Source: CAD feature listing. Evaluate the final solid. Frame: model axes, mm. Face numbers are marked on the shaded views. A direction names the side the tool comes from. Give positions to 0.01 mm unless a question says otherwise; leave off trailing zeros. Loops run counter-clockwise (first coordinate to the right, second up) from the corner with the lowest first, then second, coordinate; pieces in that order, holes last. Notation, with made-up numbers: M -33.5,72 L -21.5,72 A29 ccw -21.5,104 Z; hole C -13,52 d7. An arc over 180 degrees is marked long. Put each result on its own line as item: value. Start each with the question number.
Autodesk Inventor part; units mm, degrees
ref_plane "bolt_to_parts_XY" through (0, 0, 0) normal (1, 0, 0) x (0, 0, -1)
ref_plane "bolt_to_parts_YZ" through (0, 0, 0) normal (0, 0, -1) x (0, 1, 0)
ref_plane "bolt_to_parts_ZX" through (0, 0, 0) normal (0, 1, 0) x (1, 0, 0)
sketch "Sketch_1" plane through (0, 0, 0) normal (0, 0, 1) x (1, 0, 0)
  line L0 (5, 0) -> (-2.5, 0)
  line L1 (-2.5, 0) -> (-2.5, 0.94)
  arc A0 (0, 4.7) -> (-2.5, 0.94) centre (2.1827, 0.5376) ccw
  line L2 (0, 4.7) -> (0, 2)
  line L3 (0, 2) -> (4.5705, 2)
  line L4 (4.5705, 2) -> (5, 1.5705)
  line L5 (5, 1.5705) -> (5, 0)
  line L6 (5, 0) -> (-2.5, 0)
revolve "Revolution1" add sketch "Sketch_1" angle 360 about axis through (5, 0, 0) along (1, 0, 0)
thread "Thread1"
sketch "Sketch_2" plane through (-2.5, 0, 0) normal (1, 0, 0) x (0, 0, -1)
  line L0 (-2.35, 0.6267) -> (-2.35, -0.6267)
  line L1 (-2.35, -0.6267) -> (-0.6267, -0.6267)
  line L2 (-0.6267, -0.6267) -> (-0.6267, -2.35)
  line L3 (-0.6267, -2.35) -> (0.6267, -2.35)
  line L4 (0.6267, -2.35) -> (0.6267, -0.6267)
  line L5 (0.6267, -0.6267) -> (2.35, -0.6267)
  line L6 (2.35, -0.6267) -> (2.35, 0.6267)
  line L7 (2.35, 0.6267) -> (0.6267, 0.6267)
  line L8 (0.6267, 0.6267) -> (0.6267, 2.35)
  line L9 (0.6267, 2.35) -> (-0.6267, 2.35)
  line L10 (-0.6267, 2.35) -> (-0.6267, 0.6267)
  line L11 (-0.6267, 0.6267) -> (-2.35, 0.6267)
extrude "Extrusion1" cut sketch "Sketch_2" along normal mid plane 2.5
ref_plane "bolt_to_parts_XY" through (0, 0, 0) normal (1, 0, 0) x (0, 0, -1)
ref_plane "bolt_to_parts_YZ" through (0, 0, 0) normal (0, 0, -1) x (0, 1, 0)
ref_plane "bolt_to_parts_ZX" through (0, 0, 0) normal (0, 1, 0) x (1, 0, 0)
properties part number "BOX-TRSS4-5"
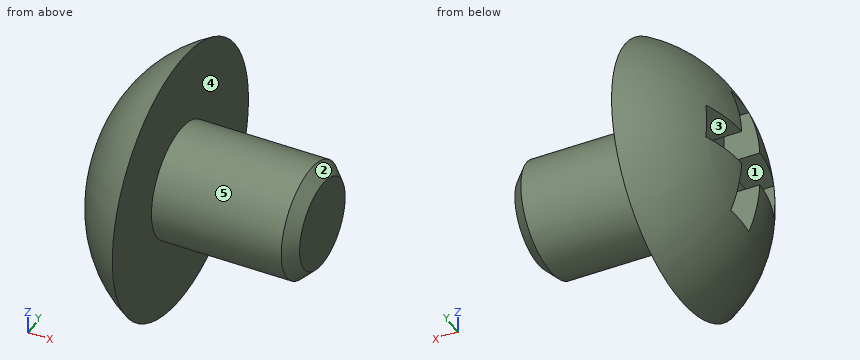
1. Section A-A, the plane x = 3. Output: boundary loops of the cut face in (y, z).
2. Ray query, line 1 (X direction, y = 1.25, z = 2); line 2 (X direction, y = 0, z = -0.5); line 3 (Z direction, x = 3.5, y = -0.25). Return the intervals inside material, ascending.
3. Set-up query: the marked faces 1 and 2. Return all of +Z, -Z, +X, -X, +Y, -Y with unobstructed straight access to the full face (end or side cutting, diameter ignored); none if empty.
4. Pull-direction query (Z, two-part tool) for the marked faces 3, 4 and 5; classes: released by +Z, released by -Z, zero draft, split by the parting line, or undercut.
5. Contact query for flat-ended pins moving along their axis: pin 1 (0.7 mm diameter, centred on x = -1.5, y = 0, fed in from +Z); pin 2 (0.5 mm diameter, centred on x = -1.5, z = 0, fed in from +Y); pin 3 (4 mm diameter, centred on x = 0.5, y = -2.5, fed in from -Z); pin 4 (4 mm diameter, centred on y = 0.5, z = 0, fed in from -X). Output: stop coordinate, or through.
Results found:
1. outline: C 0,0 d4
2. line 1: -2.15 to 0
2. line 2: -1.25 to 5
2. line 3: -1.98 to 1.98
3. face 1: -X
3. face 2: +X
4. face 3: undercut
4. face 4: zero draft
4. face 5: split by the parting line
5. pin 1: z = 3.85
5. pin 2: y = 3.75
5. pin 3: z = -4.67
5. pin 4: x = -2.5
